Work out the finished part from the listing and answer in its coordinate system (mm). Give positions to 0.01 mm unless a question says otherwise; leave off trailing zeros. Loops run counter-clockwise (first coordinate to the right, second up) from the corner with the lowest first, then second, coordinate; pieces in that order, holes last. Notation, with made-up numbers: (-24.75, -33) - (15.25, -33) arc R29 ccw to (15.25, -10) - close; hole circle Ø1 at (-12.75, 87.5). An arc over 180 degrees is marked (long way). Use one line per item in the form item = value. Start each with the question number.
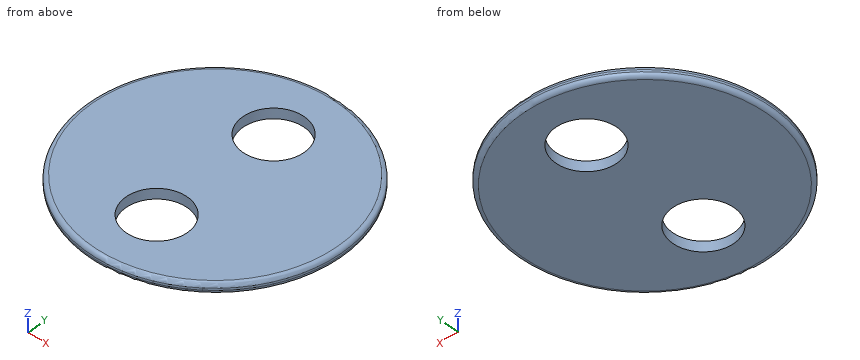
from build123d import *

# Parameters (mm, degrees)
SKETCH2_R           = 39.37
SKETCH2_R_2         = 9.525
BOSS_EXTRUDE2_DEPTH = 3.175
FILLET1_R           = 1.27


with BuildPart() as part:
    # Sketch2 → Boss-Extrude2 (new body)
    with BuildSketch(Plane.XY):
        Circle(SKETCH2_R)
        with Locations((0, 19.685)):
            Circle(SKETCH2_R_2, mode=Mode.SUBTRACT)
        with Locations((0, -19.685)):
            Circle(SKETCH2_R_2, mode=Mode.SUBTRACT)
    extrude(amount=BOSS_EXTRUDE2_DEPTH)

    # Fillet1
    fillet1_edges = [part.edges().sort_by_distance(p)[0] for p in [
        (-39.37, 0, 0),
        (-39.37, 0, 3.175),
    ]]
    fillet(fillet1_edges, radius=FILLET1_R)


solid = part.part
1) Flat-ended cylindrical pins translate along their axes: pin 1 Ø22 at (x, y) = (0, -19.685) entering from +Z (3 decimals); pin 2 Ø1 at (x, z) = (2.5, 1.5) entering from -Y; pin 3 Ø1 at (y, z) = (-9.5, 2) entering from -X; pin 4 Ø1 at (y, z) = (4.5, 2) entering from -X. Find the tip coordinate at first contact, or state that the pin passes through.
2) A cutting plane is placed at A-A (x = 0). Give the vertices of the cut face in (y, z) (3 decimals).
3) A cutting plane is placed at B-B (z = 0.6). Give the vertices of the cut face in (x, y) (3 decimals), plus the area to 3 significant figures.
4) Find the intervals of material crossed by probe 1 along Y at (x, z) = (0, 2); probe 2 along Y at (x, z) = (0, 0.8); probe 3 along X at (y, z) = (-27.5, 1.2), in increasing order.
Answer sheet:
q1.pin_1 = 3.175
q1.pin_2 = -39.32
q1.pin_3 = -38.33
q1.pin_4 = -39.17
q2.outline = (-39.37, 1.27) arc R1.27 ccw to (-38.1, 0) - (-29.21, 0) - (-29.21, 3.175) - (-38.1, 3.175) arc R1.27 ccw to (-39.37, 1.905) - close; (-10.16, 0) - (10.16, 0) - (10.16, 3.175) - (-10.16, 3.175) - close; (29.21, 0) - (38.1, 0) arc R1.27 ccw to (39.37, 1.27) - (39.37, 1.905) arc R1.27 ccw to (38.1, 3.175) - (29.21, 3.175) - close
q3.outline = circle Ø78.358 at (0, 0); hole circle Ø19.05 at (0, -19.685); hole circle Ø19.05 at (0, 19.685)
q3.area = 4,250 mm²
q4.probe_1 = -39.37 to -29.21, -10.16 to 10.16, 29.21 to 39.37
q4.probe_2 = -39.28 to -29.21, -10.16 to 10.16, 29.21 to 39.28
q4.probe_3 = -28.17 to -5.45, 5.45 to 28.17
